Check sheet for the modelled part. Datum: model origin and axes. Units: mm. A direction names the side the tool comes from. Give positions to 0.01 mm unless a question says otherwise; leave off trailing zeros. Write each loop counter-clockwise with the first axis right and the second up, starting at its lowest first coordinate (ties: lowest second). Pieces come first, ordered by that corner, then holes. Notation, with made-up numbers: (37, -7.75) -> (63, -7.75) arc R13 ccw to (63, 5.25) -> close; hole circle Ø6 at (16, 10). An arc over 180 degrees is marked (long way). Write each question's results on one line, items separated by ' | '. Start each with the question number.
```python
from build123d import *

# Parameters (mm, degrees)
F1_DEPTH = 12.7
F3_DEPTH = 12.7
F5_DEPTH = 12.7


with BuildPart() as f1:
    # F0 (on Top) → F1 (new body)
    with BuildSketch(Plane.XY):
        Polygon((-57.260543, -47.510773), (-37.141975, -47.510773), (55.093925, -47.510773), (55.093925, 29.868338), (-57.260543, 29.868338), align=None)
    extrude(amount=F1_DEPTH)

    # F2 (on face) → F3 (join)
    with BuildSketch(Plane.XY.offset(12.7)):
        Polygon((-43.641821, -47.510773), (-12.99969, 29.868338), (-57.260543, 29.868338), (-57.260543, -47.510773), align=None)
    extrude(amount=F3_DEPTH)

    # F4 (on face) → F5 (join)
    with BuildSketch(Plane.XY.offset(12.7)):
        Polygon((55.093925, -22.749459), (35.284877, -47.510773), (55.093925, -47.510773), align=None)
    extrude(amount=F5_DEPTH)


solid = f1.part
```
Item 1: Section check A-A on z = 18.75. Record the boundary of the cut face in (x, y).
Item 2: Section check C-C on x = -7.5. Record the boundary of the cut face in (y, z), then the cut area to 3 significant figures.
Item 3: Section check B-B on y = -37.5. Record the boundary of the cut face in (x, z), then the cut area to 3 significant figures.
Item 4: Depth check by flat-ended pin: pin 1 Ø4 at (x, y) = (17, 21.5) entering from +Z. Enter the tip coordinate at first touch or a pass-through.
Item 5: Section check D-D on y = -29.5. Record the boundary of the cut face in (x, z), then the cut area to 3 significant figures.
Item 6: Thickness scan on probe 1 along Z at (x, y) = (13, 5); probe 2 along X at (y, z) = (-35.5, 19.75); probe 3 along X at (y, z) = (-44, 22.25). Record the ranges inside material, lowest first. Write a range as from..to.
Item 7: Mould release check, pull along X, two halves, no side actions. Record for faces 4 (the flat face through (16, -8, 12.7)), 5 (the flat face through (-57.261, -8, 13)), 6 (the flat face through (-2, -8, 0)): pulls with the +X half, pulls with the -X half, needs draft (parallel to the pull), parting line crosses it, or undercut.
Item 8: Set-up check for faces 1 (the flat face through (49, -40, 25.4)), 2 (the flat face through (45.328, -34.957, 18.961)), 3 (the flat face through (-28.535, -9.363, 18.961)): record each of +Z, -Z, +X, -X, +Y, -Y from which the full face is reachable in a straight line by a thin tool's end or side.
Check sheet entries:
1) outline: (-57.26, -47.51) -> (-43.64, -47.51) -> (-13, 29.87) -> (-57.26, 29.87) -> close; (35.28, -47.51) -> (55.09, -47.51) -> (55.09, -22.75) -> close
2) outline: (-47.51, 0) -> (29.87, 0) -> (29.87, 12.7) -> (-47.51, 12.7) -> close | area: 983 mm^2
3) outline: (-57.26, 0) -> (55.09, 0) -> (55.09, 25.4) -> (43.29, 25.4) -> (43.29, 12.7) -> (-39.68, 12.7) -> (-39.68, 25.4) -> (-57.26, 25.4) -> close | area: 1,800 mm^2
4) pin 1: stops at z = 12.7
5) outline: (-57.26, 0) -> (55.09, 0) -> (55.09, 25.4) -> (49.69, 25.4) -> (49.69, 12.7) -> (-36.51, 12.7) -> (-36.51, 25.4) -> (-57.26, 25.4) -> close | area: 1,760 mm^2
6) probe 1: z = 0..12.7 | probe 2: x = -57.26..-38.89, 44.89..55.09 | probe 3: x = -57.26..-42.25, 38.09..55.09
7) face 4: undercut | face 5: pulls with the -X half | face 6: needs draft
8) face 1: +Z, +X, -X, +Y, -Y | face 2: +Z, +Y | face 3: +Z, -Y
